```python
from build123d import *

# Parameters (mm, degrees)
SKETCH_1_R          = 3
EXTRUDE_1_DEPTH     = 0.5
SKETCH_2_R          = 1.5
EXTRUDE_2_DEPTH     = 5
CHAMFER_1_SIZE      = 0.2
CUT_EXTRUDE_1_DEPTH = 0.8
FILLET_2_R          = 0.3


with BuildPart() as part:
    # 草图1 → 凸台-拉伸1 (new body, symmetric)
    with BuildSketch(Plane.XY):
        Circle(SKETCH_1_R)
    extrude(amount=EXTRUDE_1_DEPTH, both=True)

    # 草图2 → 凸台-拉伸2 (add)
    with BuildSketch(Plane(origin=(0, 0, -0.5), x_dir=(-1, 0, 0), z_dir=(0, 0, -1))):
        Circle(SKETCH_2_R)
    extrude(amount=EXTRUDE_2_DEPTH)

    # 倒角1
    chamfer_1_edges = [part.edges().sort_by_distance(p)[0] for p in [
        (1.5, 0, -5.5),
    ]]
    chamfer(chamfer_1_edges, length=CHAMFER_1_SIZE)

    # 草图3 → 切除-拉伸1 (cut)
    with BuildSketch(Plane.XY.offset(0.5)):
        Polygon((1.154700538, 0), (0.577350269, 1), (-0.577350269, 1), (-1.154700538, 0), (-0.577350269, -1), (0.577350269, -1), align=None)
    extrude(amount=-CUT_EXTRUDE_1_DEPTH, mode=Mode.SUBTRACT)

    # 圆角2
    fillet_2_edges = [part.edges().sort_by_distance(p)[0] for p in [
        (-3, 0, -0.5),
        (-3, 0, 0.5),
    ]]
    fillet(fillet_2_edges, radius=FILLET_2_R)


solid = part.part
```
The model under review builds one solid part; all positions refer to its coordinate system, in mm. A direction names the side the tool comes from. Give positions to 0.01 mm unless a question says otherwise; leave off trailing zeros. Write each loop counter-clockwise with the first axis right and the second up, starting at its lowest first coordinate (ties: lowest second). Pieces come first, ordered by that corner, then holes. Notation, with made-up numbers: (76, 48) - (102, 48) arc R23 cw to (102, 69) - close; hole circle Ø1 at (-11.5, -25). An arc over 180 degrees is marked (long way). Answer in a Markdown table with one row per item. Add a question column.
1. We need section B-B on z = 0. Write out the cut boundary in (x, y).
2. We need section A-A on x = 0. Write out the cut boundary in (y, z), then the cut area to 3 significant figures.
3. Wall thickness on line 1 along Z through (x, y) = (0.75, 1.5); line 2 along Z through (x, y) = (1, 0); line 3 along X through (y, z) = (-0.75, -1.9): over which ranges is each line inside the solid? List them lowest first. Write a range as [from, to].
4. Insertion check: P1, Ø2, axis at x = 1.5, z = -1, coming from the -Y side; P2, Ø1.6, axis at x = 0, y = 0, coming from the +Z side. Each pin has a flat end and moves straight along its axis. Give the tip position at first contact, or say it passes through.
5. We need section C-C on z = -4.85. Write out the cut boundary in (x, y).
6. Draft analysis for pull direction X (two halves, no side actions). For faces 1 (the cylindrical face through (-3, 0, 0)), 2 (the flat face through (0, 0, -5.5)), 3 (the flat face through (0, 0, -0.3)), state which applies: +X half, -X half, draft (parallel to the pull), parting line (faces both ways), or undercut.
7. Tool access review of faces 4 (the flat face through (0, -1.2, 0.5)), 5 (the flat face through (1.2, -1.2, -0.5)): name each direction out of +Z, -Z, +X, -X, +Y, -Y from which nothing blocks a thin tool from reaching the whole face with its end or side.
Ans:
| question | item | result |
|---|---|---|
| 1 | outline | circle Ø6 at (0, 0); hole (-1.15, 0) - (-0.58, -1) - (0.58, -1) - (1.15, 0) - (0.58, 1) - (-0.58, 1) - close |
| 2 | outline | (-3, -0.2) arc R0.3 ccw to (-2.7, -0.5) - (-1.5, -0.5) - (-1.5, -5.3) - (-1.3, -5.5) - (1.3, -5.5) - (1.5, -5.3) - (1.5, -0.5) - (2.7, -0.5) arc R0.3 ccw to (3, -0.2) - (3, 0.2) arc R0.3 ccw to (2.7, 0.5) - (1, 0.5) - (1, -0.3) - (-1, -0.3) - (-1, 0.5) - (-2.7, 0.5) arc R0.3 ccw to (-3, 0.2) - close |
| 2 | area | 19.3 mm^2 |
| 3 | line 1 | z = [-0.5, 0.5] |
| 3 | line 2 | z = [-5.5, -0.3] |
| 3 | line 3 | x = [-1.3, 1.3] |
| 4 | P1 | stops at y = -2.88 |
| 4 | P2 | stops at z = -0.3 |
| 5 | outline | circle Ø3 at (0, 0) |
| 6 | face 1 | parting line |
| 6 | face 2 | draft |
| 6 | face 3 | undercut |
| 7 | face 4 | +Z, +X, -X, +Y, -Y |
| 7 | face 5 | -Z |
